from build123d import *
from OCP.BRepFilletAPI import BRepFilletAPI_MakeFillet

# Parameters (mm, degrees)
SKETCH1_R           = 2.5
BOSS_EXTRUDE1_DEPTH = 3
FILLET1_R1          = 10
FILLET1_R2          = 15
FILLET1_R3          = 20
SKETCH2_R           = 1.75
SKETCH2_R_2         = 12
CUT_EXTRUDE1_DEPTH  = 45.331140297


with BuildPart() as part:
    # Sketch1 → Boss-Extrude1 (new body)
    with BuildSketch(Plane.XY):
        Polygon((-32.5, 30), (32.5, 30), (32.5, -10), (0, -35), (-32.5, -10), align=None)
        with Locations((25, 20)):
            Circle(SKETCH1_R, mode=Mode.SUBTRACT)
        with Locations((-25, 20)):
            Circle(SKETCH1_R, mode=Mode.SUBTRACT)
        with BuildLine():
            Line((2.5, -16.5), (2.5, -23.5))
            ThreePointArc((2.5, -23.5), (0, -26), (-2.5, -23.5))
            Line((-2.5, -23.5), (-2.5, -16.5))
            ThreePointArc((-2.5, -16.5), (0, -14), (2.5, -16.5))
        make_face(mode=Mode.SUBTRACT)
    extrude(amount=BOSS_EXTRUDE1_DEPTH)

    # Fillet1: one fillet with a radius per group of edges: ONE call of the kernel's fillet builder (fillet() takes one radius for all edges)
    fillet1_edges_1 = [part.edges().sort_by_distance(p)[0] for p in [
        (32.5, 30, 1.5),
        (-32.5, 30, 1.5),
    ]]
    fillet1_edges_2 = [part.edges().sort_by_distance(p)[0] for p in [
        (-32.5, -10, 1.5),
        (32.5, -10, 1.5),
    ]]
    fillet1_edges_3 = [part.edges().sort_by_distance(p)[0] for p in [
        (0, -35, 1.5),
    ]]
    fillet1 = BRepFilletAPI_MakeFillet(part.part.solid().wrapped)
    for e in fillet1_edges_1:
        fillet1.Add(FILLET1_R1, e.wrapped)
    for e in fillet1_edges_2:
        fillet1.Add(FILLET1_R2, e.wrapped)
    for e in fillet1_edges_3:
        fillet1.Add(FILLET1_R3, e.wrapped)
    add(Compound.cast(fillet1.Shape()), mode=Mode.REPLACE)

    # Sketch2 → Cut-Extrude1 (cut, through all)
    with BuildSketch(Plane.XY.offset(3)):
        with Locations((12, 7)):
            Circle(SKETCH2_R)
        with Locations((12, -17)):
            Circle(SKETCH2_R)
        with Locations((-12, -17)):
            Circle(SKETCH2_R)
        with Locations((-12, 7)):
            Circle(SKETCH2_R)
        with Locations((0, -5)):
            Circle(SKETCH2_R_2)
    extrude(amount=-CUT_EXTRUDE1_DEPTH, mode=Mode.SUBTRACT)


solid = part.part
Can you work these out from the model? Positions are in its coordinate system, mm. A direction names the side the tool comes from. Give positions to 0.01 mm unless a question says otherwise; leave off trailing zeros. Loops run counter-clockwise (first coordinate to the right, second up) from the corner with the lowest first, then second, coordinate; pieces in that order, holes last. Notation, with made-up numbers: (72, 7.5) -> (115, 7.5) arc R12 ccw to (115, 14.5) -> close; hole circle Ø4 at (-40, 84). An arc over 180 degrees is marked (long way). Return JSON: item names as keys, results as strings.
Q1. We'd pull the mould along Y, two halves only. Please class faces 1 (the face through (29.49, 27.15, 1.52)), 2 (the face through (-26.84, 21.69, 1.48)), 3 (the face through (-32.5, 9, 1)): released by +Y, released by -Y, zero draft, split by the parting line, or undercut.
Checks:
{"face 1": "released by +Y", "face 2": "undercut", "face 3": "zero draft"}
Q2. For pin 1 Ø0.9 at (y, z) = (-21, 1.5) entering from -X (3 decimals), with a flat end and sliding along its axis, tell me the tip position at first contact or that it passes through.
Checks:
{"pin 1": "stops at x = -18.785"}
Q3. I need wall thicknesses on probe 1 along X at (y, z) = (8, 1.1); probe 2 along X at (y, z) = (8.5, 2.7); probe 3 along Y at (x, z) = (0, 1.3). Which ranges of each line are inside material? Lowest first, please.
Checks:
{"probe 1": "x = -32.5 to -13.44, -10.56 to 10.56, 13.44 to 32.5", "probe 2": "x = -32.5 to -12.9, -11.1 to 11.1, 12.9 to 32.5", "probe 3": "y = -29.77 to -26, 7 to 30"}
Q4. I want a section at D-D, the plane x = 16. List the corners of the cut face in (y, z) for me, then the cut area to 3 significant figures.
Checks:
{"outline": "(-22.69, 0) -> (30, 0) -> (30, 3) -> (-22.69, 3) -> close", "area": "158 mm2"}
Q5. I want a section at A-A, the plane x = 0. List the corners of the cut face in (y, z) for me, then the cut area to 3 significant figures.
Checks:
{"outline": "(-29.77, 0) -> (-26, 0) -> (-26, 3) -> (-29.77, 3) -> close; (7, 0) -> (30, 0) -> (30, 3) -> (7, 3) -> close", "area": "80.3 mm2"}
Q6. I want a section at C-C, the plane y = -5. List the corners of the cut face in (x, z) for me.
Checks:
{"outline": "(-32.31, 0) -> (-12, 0) -> (-12, 3) -> (-32.31, 3) -> close; (12, 0) -> (32.31, 0) -> (32.31, 3) -> (12, 3) -> close"}
Q7. I want a section at B-B, the plane z = 2.2. List the corners of the cut face in (x, y) for me, then the cut area to 3 significant figures.
Checks:
{"outline": "(-32.5, -2.61) arc R15 ccw to (-26.65, -14.5) -> (-12.19, -25.62) arc R20 ccw to (12.19, -25.62) -> (26.65, -14.5) arc R15 ccw to (32.5, -2.61) -> (32.5, 20) arc R10 ccw to (22.5, 30) -> (-22.5, 30) arc R10 ccw to (-32.5, 20) -> close; hole circle Ø5 at (-25, 20); hole circle Ø3.5 at (-12, -17); hole circle Ø3.5 at (-12, 7); hole (-2.5, -23.5) arc R2.5 ccw to (2.5, -23.5) -> (2.5, -16.74) arc R12 ccw (long way) to (-2.5, -16.74) -> close; hole circle Ø3.5 at (12, -17); hole circle Ø3.5 at (12, 7); hole circle Ø5 at (25, 20)", "area": "2,740 mm2"}
Q8. On a 3-axis mill with a long thin cutter (end or side, diameter ignored), from which of +Z, -Z, +X, -X, +Y, -Y can I reach the whole of each face in a straight line? I mean faces 4 (the face through (19.5, -20, 1.5)), 5 (the face through (-2.5, -20, 1)). Say none if no direction works.
Checks:
{"face 4": "+Z, -Z, +X, -Y", "face 5": "+Z, -Z"}
